Study the drawing (mm; zero at the part's minimum x, y, z) and answer. A direction names the side the tool comes from. Coordinates: 2 decimals unless noted, no trailing zeros. Loops run counter-clockwise (first coordinate to the right, second up) from the corner with the lowest first, then second, coordinate; pieces in that order, holes last. Notation, with made-up numbers: (70.5, 9.5) - (91.5, 9.5) arc R15 ccw to (91.5, 13.5) - close; hole circle Ø5 at (58, -18). An arc over 180 degrees is marked (long way). Put each result on its own line as item: value.
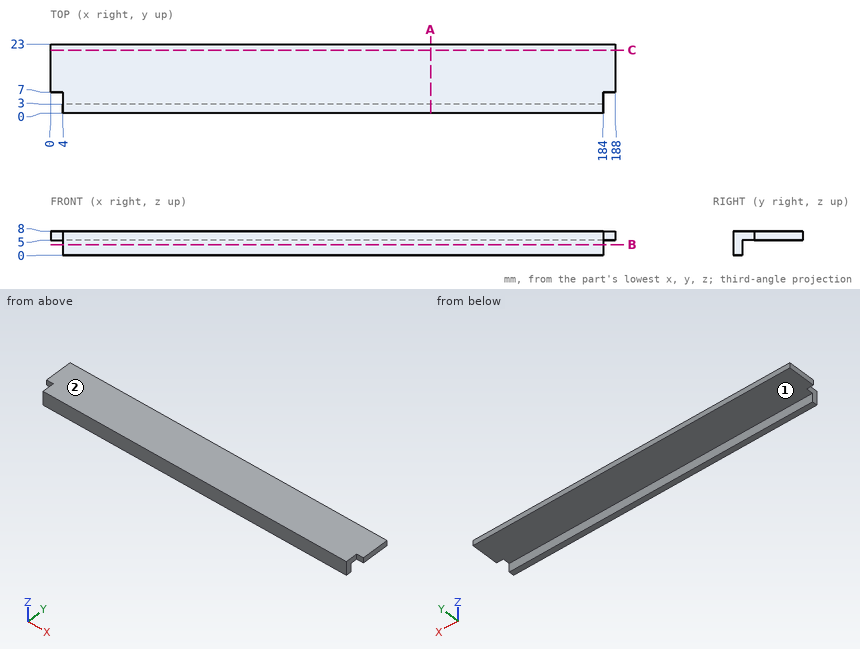
1) For the marked faces 1 and 2, determine the directions among +Z, -Z, +X, -X, +Y, -Y from which every point of the face is accessible in a straight line to the end or side of a thin tool.
Found:
face 1: -Z, +X, -X, +Y
face 2: +Z, +X, -X, +Y, -Y
2) The part is cut by section B-B (z = 3.5). Give the vertices of the cut face in (x, y), and give its area (3 significant figures).
Found:
outline: (4, 0) - (184, 0) - (184, 3) - (4, 3) - close
area: 540 mm^2
3) Straight lines are drawn through the part: L1, parallel to Y at x = 17.5, z = 3; L2, parallel to Z at x = 133, y = 21.5; L3, parallel to X at y = 5.5, z = 6. For each, find the intervals that lie inside material, in ascending order. Write a range as [from, to].
Found:
L1: y = [0, 3]
L2: z = [5, 8]
L3: x = [4, 184]
4) Each of these flat-tipped pins is pushed along its axis until it touches: pin 1 (3.5 mm diameter, centred on y = 4, z = 3, fed in from +X); pin 2 (0.9 mm diameter, centred on x = 185.5, z = 6, fed in from -Y); pin 3 (6 mm diameter, centred on x = 90.5, y = 16, fed in from -Z). Where does it stop, or does it pass through?
Found:
pin 1: stops at x = 184
pin 2: stops at y = 7
pin 3: stops at z = 5
5) The part is cut by section C-C (y = 21). Give the vertices of the cut face in (x, z), and give its area (3 significant figures).
Found:
outline: (0, 5) - (188, 5) - (188, 8) - (0, 8) - close
area: 564 mm^2
6) The part is cut by section A-A (x = 126.5). Give the vertices of the cut face in (y, z), and give its area (3 significant figures).
Found:
outline: (0, 0) - (3, 0) - (3, 5) - (23, 5) - (23, 8) - (0, 8) - close
area: 84.0 mm^2
